from build123d import *

# Parameters (mm, degrees)
SKETCH1_W                 = 393.7
SKETCH1_H                 = 457.2
PLATE_DEPTH               = 12.7
PATTERN_LINEAR_1110_COUNT = 4
PATTERN_LINEAR_1110_PITCH = 127


with BuildPart() as part:
    # Sketch1 → Plate (new body)
    with BuildSketch(Plane.XY):
        with Locations((196.85, 228.6)):
            Rectangle(SKETCH1_W, SKETCH1_H)
    extrude(amount=PLATE_DEPTH)

    # Sketch3 → Hole (revolve, cut)
    with BuildSketch(Plane(origin=(44.45, 38.1, 12.7), x_dir=(0, -1, 0), z_dir=(1, 0, 0))):
        Polygon((0, 0), (0, 29.215464931), (6.35, 25.4), (6.35, 0), align=None)
    hole = revolve(axis=Axis((44.45, 38.1, 19.05), (0, 0, -1)), mode=Mode.SUBTRACT)

    # Pattern Linear 1110: Hole ×4
    with Locations(*[(0, i * PATTERN_LINEAR_1110_PITCH, 0) for i in range(1, PATTERN_LINEAR_1110_COUNT)]):
        add(hole, mode=Mode.SUBTRACT)


solid = part.part
Source: CAD feature listing. Evaluate the final solid. Frame: model axes, mm. Give positions to 0.01 mm unless a question says otherwise; leave off trailing zeros. Write each loop counter-clockwise with the first axis right and the second up, starting at its lowest first coordinate (ties: lowest second). Pieces come first, ordered by that corner, then holes. Notation, with made-up numbers: (59.5, 15) -> (109.5, 15) arc R27 ccw to (109.5, 52) -> close; hole circle Ø4 at (19.5, 67.5). An arc over 180 degrees is marked (long way). Return JSON: item names as keys, results as strings. Group by question number.
1. Section B-B, the plane y = 419.1. Output: boundary loops of the cut face in (x, z), then the cut area to 3 significant figures.
2. Section A-A, the plane x = 44.45. Output: boundary loops of the cut face in (y, z).
3. Material intervals for line 1 (Y direction, x = 44.45, z = 4.5); line 2 (X direction, y = 38.1, z = 4), sorted ascending. Write a range as from..to.
4. Mould query, pull axis X, two halves, no side actions, for faces 1 (the face through (0, 225, 6)), 2 (the face through (42.543, 159.043, 6.439)), 3 (the face through (194, 0, 6)). Classes: +X half, -X half, draft (parallel to the pull), parting line (faces both ways), or undercut.
Determined:
{
 "1": {"outline": "(0, 0) -> (38.1, 0) -> (38.1, 12.7) -> (0, 12.7) -> close; (50.8, 0) -> (393.7, 0) -> (393.7, 12.7) -> (50.8, 12.7) -> close", "area": "4,840 mm2"},
 "2": {"outline": "(0, 0) -> (31.75, 0) -> (31.75, 12.7) -> (0, 12.7) -> close; (44.45, 0) -> (158.75, 0) -> (158.75, 12.7) -> (44.45, 12.7) -> close; (171.45, 0) -> (285.75, 0) -> (285.75, 12.7) -> (171.45, 12.7) -> close; (298.45, 0) -> (412.75, 0) -> (412.75, 12.7) -> (298.45, 12.7) -> close; (425.45, 0) -> (457.2, 0) -> (457.2, 12.7) -> (425.45, 12.7) -> close"},
 "3": {"line 1": "y = 0..31.75, 44.45..158.75, 171.45..285.75, 298.45..412.75, 425.45..457.2", "line 2": "x = 0..38.1, 50.8..393.7"},
 "4": {"face 1": "-X half", "face 2": "undercut", "face 3": "draft"}
}
